Read the model definition and answer for the solid it produces. Units are mm, in the model's axes. A direction names the side the tool comes from. Give positions to 0.01 mm unless a question says otherwise; leave off trailing zeros. Write each loop counter-clockwise with the first axis right and the second up, starting at its lowest first coordinate (ties: lowest second). Pieces come first, ordered by that corner, then holes. Notation, with made-up numbers: (89, 19) - (132, 19) arc R25 cw to (132, 50) - close; hole circle Ø5 at (-34.5, 14). An arc over 180 degrees is marked (long way). Answer as CSV lines item,"result".
```python
from build123d import *

# Parameters (mm, degrees)
SKETCH1_R           = 2.5
BOSS_EXTRUDE1_DEPTH = 1.5
SKETCH2_R           = 14
SKETCH2_R_2         = 2.5
BOSS_EXTRUDE2_DEPTH = 3
SKETCH4_R           = 1.5
SKETCH4_R_2         = 2.502
BOSS_EXTRUDE3_DEPTH = 1.5
SKETCH3_R           = 2
CUT_EXTRUDE1_DEPTH  = 7.5
SKETCH5_R           = 11
SKETCH5_R_2         = 2.5
BOSS_EXTRUDE4_DEPTH = 1


with BuildPart() as part:
    # Sketch1 → Boss-Extrude1 (new body)
    with BuildSketch(Plane(origin=(0, 0, 0), x_dir=(0, 0, -1), z_dir=(1, 0, 0))):
        with BuildLine():
            Line((-16, 22), (16, 22))
            ThreePointArc((16, 22), (20.242640687, 20.242640687), (22, 16))
            Line((22, 16), (22, -16))
            ThreePointArc((22, -16), (20.242640687, -20.242640687), (16, -22))
            Line((16, -22), (-16, -22))
            ThreePointArc((-16, -22), (-20.242640687, -20.242640687), (-22, -16))
            Line((-22, -16), (-22, 16))
            ThreePointArc((-22, 16), (-20.242640687, 20.242640687), (-16, 22))
        make_face()
        Circle(SKETCH1_R, mode=Mode.SUBTRACT)
    extrude(amount=BOSS_EXTRUDE1_DEPTH)

    # Sketch2 → Boss-Extrude2 (add)
    with BuildSketch(Plane(origin=(1.5, 0, 0), x_dir=(0, 0, -1), z_dir=(1, 0, 0))):
        Circle(SKETCH2_R)
        Circle(SKETCH2_R_2, mode=Mode.SUBTRACT)
    extrude(amount=BOSS_EXTRUDE2_DEPTH)

    # Sketch4 → Boss-Extrude3 (add)
    with BuildSketch(Plane(origin=(4.5, 0, 0), x_dir=(0, 0, -1), z_dir=(1, 0, 0))):
        with BuildLine():
            Line((-3.723678165, 17.610205059), (14.314456464, 21.426417539))
            ThreePointArc((14.314456464, 21.426417539), (19.79871712, 19.799262609), (21.426577165, 14.315211208))
            Line((21.426577165, 14.315211208), (17.612683935, -3.723413935))
            ThreePointArc((17.612683935, -3.723413935), (12.730477998, -12.7273661), (3.726952372, -17.610358594))
            Line((3.726952372, -17.610358594), (-14.314460707, -21.426487839))
            ThreePointArc((-14.314460707, -21.426487839), (-19.798989873, -19.798771294), (-21.426091866, -14.314059778))
            Line((-21.426091866, -14.314059778), (-17.607941103, 3.726925591))
            ThreePointArc((-17.607941103, 3.726925591), (-12.725471256, 12.728372851), (-3.723678165, 17.610205059))
        make_face()
        with Locations((15.556349186, 15.556349186)):
            Circle(SKETCH4_R, mode=Mode.SUBTRACT)
        with Locations((-15.554349186, -15.556349186)):
            Circle(SKETCH4_R, mode=Mode.SUBTRACT)
        with Locations(Location((0.002, 0, 0), (0, 0, 180))):
            Circle(SKETCH4_R_2, mode=Mode.SUBTRACT)
    extrude(amount=BOSS_EXTRUDE3_DEPTH)

    # Sketch3 → Cut-Extrude1 (cut)
    with BuildSketch(Plane(origin=(4.5, 0, 0), x_dir=(0, 0, -1), z_dir=(1, 0, 0))):
        with Locations((15.556349186, 15.556349186)):
            Circle(SKETCH3_R)
        with Locations((15.556349186, -15.556349186)):
            Circle(SKETCH3_R)
        with Locations((-15.556349186, -15.556349186)):
            Circle(SKETCH3_R)
        with Locations((-15.556349186, 15.556349186)):
            Circle(SKETCH3_R)
    extrude(amount=-CUT_EXTRUDE1_DEPTH, mode=Mode.SUBTRACT)

    # Sketch5 → Boss-Extrude4 (add)
    with BuildSketch(Plane(origin=(6, 0, 0), x_dir=(0, 0, -1), z_dir=(1, 0, 0))):
        Circle(SKETCH5_R)
        with Locations(Location((0, 0, 0), (0, 0, 180))):
            Circle(SKETCH5_R_2, mode=Mode.SUBTRACT)
    extrude(amount=BOSS_EXTRUDE4_DEPTH)


solid = part.part
```
(1) The mould has two halves that part along Y. Classify faces 1 (the flat face through (1, 0, -22)), 2 (the cylindrical face through (0.8, 14.3, -14)), 3 (the cylindrical face through (0.74, 20.196, 20.289)), 4 (the cylindrical face through (5.24, -17.02, 15.88)): +Y half, -Y half, draft (parallel to the pull), parting line (faces both ways), or undercut.
Worked out:
face 1,"draft"
face 2,"undercut"
face 3,"+Y half"
face 4,"undercut"
(2) Find the intervals of material crossed by L1, parallel to X at y = 18, z = -4; L2, parallel to Z at x = 1, y = 15.5; L3, parallel to Y at x = 6.6, z = 0, in increasing order.
Worked out:
L1,"x = 0 to 1.5, 4.5 to 6"
L2,"z = -22 to -17.56, -13.56 to 13.56, 17.56 to 22"
L3,"y = -11 to -2.5, 2.5 to 11"
(3) A cutting plane is placed at A-A (y = 19). Write down the section's boundary in (x, z), and give its area (3 significant figures).
Worked out:
outline,"(0, -21.2) - (1.5, -21.2) - (1.5, 21.2) - (0, 21.2) - close; (4.5, -20.47) - (6, -20.47) - (6, -2.85) - (4.5, -2.85) - close"
area,"90.0 mm^2"
(4) A cutting plane is placed at C-C (x = 0.75). Write down the section's boundary in (y, z), and give its area (3 significant figures).
Worked out:
outline,"(-22, -16) arc R6 ccw to (-16, -22) - (16, -22) arc R6 ccw to (22, -16) - (22, 16) arc R6 ccw to (16, 22) - (-16, 22) arc R6 ccw to (-22, 16) - close; hole circle Ø4 at (-15.56, -15.56); hole circle Ø4 at (-15.56, 15.56); hole circle Ø5 at (0, 0); hole circle Ø4 at (15.56, -15.56); hole circle Ø4 at (15.56, 15.56)"
area,"1,840 mm^2"
(5) Each of these flat-tipped pins is pushed along its axis until it touches: P1, Ø4, axis at y = -15.56, z = 15.55, coming from the +X side; P2, Ø3, axis at x = 5.5, z = 7, coming from the -Y side; P3, Ø6.5, axis at y = -15.56, z = -15.56, coming from the +X side. Where does it stop, or does it pass through?
Worked out:
P1,"stops at x = 6"
P2,"stops at y = -20.2"
P3,"stops at x = 1.5"
(6) For faces 5 (the flat face through (6, 5, -10)), 6 (the cylindrical face through (2.979, -5.362, -12.932)), 7 (the cylindrical face through (0.76, -17.51, 15.99)), determine the directions among +Z, -Z, +X, -X, +Y, -Y from which every point of the face is accessible in a straight line to the end or side of a thin tool.
Worked out:
face 5,"+X"
face 6,"none"
face 7,"-X"
(7) A cutting plane is placed at D-D (y = 12.5). Write down the section's boundary in (x, z).
Worked out:
outline,"(0, -22) - (1.5, -22) - (1.5, -6.3) - (4.5, -6.3) - (4.5, -21.04) - (6, -21.04) - (6, 12.95) - (4.5, 12.95) - (4.5, 6.3) - (1.5, 6.3) - (1.5, 22) - (0, 22) - close"
